Autodesk Inventor part; units mm, degrees
ref_plane "BoardFrontPlane" through (0, 0, 0) normal (0, 0, 1) x (1, 0, 0)
ref_plane "YZ Plane" through (0, 0, 0) normal (1, 0, 0) x (0, 1, 0)
ref_plane "XZ Plane" through (0, 0, 0) normal (0, 1, 0) x (-1, 0, 0)
ref_plane "BoardFrontPlane" through (0, 0, 0) normal (0, 0, 1) x (1, 0, 0)
sketch "Sketch1" plane through (0, 0, 0) normal (0, 0, 1) x (1, 0, 0)
  line L0 (35, 26) -> (35, 27)
  line L1 (35, 27) -> (75, 27)
  line L2 (75, 27) -> (75, 26)
  line L3 (75, 26) -> (83.3, 26)
  line L4 (83.3, 26) -> (83.3, 33.05)
  line L5 (83.3, 33.05) -> (128.7, 33.05)
  line L6 (128.7, 33.05) -> (128.7, 26)
  line L7 (128.7, 26) -> (147, 26)
  line L8 (147, 26) -> (147, 27)
  line L9 (147, 27) -> (171, 27)
  line L10 (171, 27) -> (171, 26)
  line L11 (171, 26) -> (186, 26)
  line L12 (186, 26) -> (186, 113)
  line L13 (186, 113) -> (128.7, 113)
  line L14 (128.7, 113) -> (128.7, 105.95)
  line L15 (128.7, 105.95) -> (83.3, 105.95)
  line L16 (83.3, 105.95) -> (83.3, 113)
  line L17 (83.3, 113) -> (26, 113)
  line L18 (26, 113) -> (26, 26)
  line L19 (26, 26) -> (35, 26)
extrude "BoardOutline" add sketch "Sketch1" along normal blind 1.5957
ref_plane "Work Plane2" through (106, 26, 0) normal (1, 0, 0) x (0, 0, -1)
ref_plane "Work Plane3" through (171, 69.5, 0) normal (0, -1, 0) x (1, 0, 0)
sketch "Sketch4" plane through (0, 0, 1.5957) normal (0, 0, 1) x (1, 0, 0)
  line L0 (83.3, 26) -> (83.3, 33.05)
  line L1 (83.3, 33.05) -> (128.7, 33.05)
  line L2 (128.7, 33.05) -> (128.7, 26)
  line L3 (26, 113) -> (26, 26)
  line L4 (83.3, 26) -> (128.7, 26)
  point P0 (83.3, 29.525)
  point P1 (186, 26)
  dimension "d9" = 57.3
  dimension "d10" = 57.3
  dimension "d11" = 7.05
sketch "Sketch8" plane through (0, 0, 1.5957) normal (0, 0, 1) x (1, 0, 0)
  point P0 (106, 94.5)
hole "Free-Hole1_1" at (106, 94.5, 1.5957) direction (0, 0, -1) diameter 3.6 end through all
sketch "Sketch9" plane through (0, 0, 1.5957) normal (0, 0, 1) x (1, 0, 0)
  point P0 (106, 44.5)
hole "Free-Hole1_2_1" at (106, 44.5, 1.5957) direction (0, 0, -1) diameter 3.6 end through all
sketch "Sketch11" plane through (0, 0, 1.5957) normal (0, 0, 1) x (1, 0, 0)
  point P0 (46, 94.5)
hole "Free-Hole4_1" at (46, 94.5, 1.5957) direction (0, 0, -1) diameter 3.6 end through all
sketch "Sketch12" plane through (0, 0, 1.5957) normal (0, 0, 1) x (1, 0, 0)
  point P0 (46, 44.5)
hole "Free-Hole4_2_1" at (46, 44.5, 1.5957) direction (0, 0, -1) diameter 3.6 end through all
sketch "Sketch13" plane through (0, 0, 1.5957) normal (0, 0, 1) x (1, 0, 0)
  point P0 (166, 44.5)
hole "Free-Hole4_3_1" at (166, 44.5, 1.5957) direction (0, 0, -1) diameter 3.6 end through all
sketch "Sketch14" plane through (0, 0, 1.5957) normal (0, 0, 1) x (1, 0, 0)
  point P0 (166, 94.5)
hole "Free-Hole4_4_1" at (166, 94.5, 1.5957) direction (0, 0, -1) diameter 3.6 end through all
sketch "img_Top" plane through (0, 0, 1.5957) normal (0, 0, 1) x (1, 0, 0)
  line L0 (26, 113) -> (186, 113) construction
  line L1 (186, 113) -> (186, 26.0021) construction
  line L2 (186, 26.0021) -> (26, 26.0021) construction
  line L3 (26, 26.0021) -> (26, 113) construction
decal "Decal_Top"
properties part number "ledbrick_plus_led_BOARD"
The listing builds one solid part. Answer for the finished solid, in the listing's coordinates (mm). Coordinates: 2 decimals unless noted, no trailing zeros. Write each loop counter-clockwise with the first axis right and the second up, starting at its lowest first coordinate (ties: lowest second). Pieces come first, ordered by that corner, then holes. Notation, with made-up numbers: (-38.75, 78) -> (-24.75, 78) arc R17 cw to (-24.75, 84) -> close; hole circle Ø4 at (72.25, 30.25). An arc over 180 degrees is marked (long way). Write each question's results on one line, items separated by ' | '. Start each with the question number.
1) For a pull along Y with two mould halves and no side action, classify faces 1 (the cylindrical face through (167.757, 94.89, 0.787)), 2 (the flat face through (105, 70, 1.596)) as +Y half, -Y half, draft (parallel to the pull), parting line (faces both ways), or undercut.
2) A cutting plane is placed at A-A (x = 166). Determine the outline of the cut face in (y, z).
3) A cutting plane is placed at D-D (x = 106). Determine the outline of the cut face in (y, z).
4) A cutting plane is placed at B-B (z = 0.4). Determine the outline of the cut face in (x, y), then the cut area to 3 significant figures.
5) Straight lines are drawn through the part: probe 1 along X at (y, z) = (94.5, 0.55); probe 2 along Y at (x, z) = (106, 1.1); probe 3 along Y at (x, z) = (46, 1.15). For each, find the intervals that lie inside material, in ascending order.
6) A cutting plane is placed at C-C (y = 44.5). Determine the outline of the cut face in (x, z).
7) Flat-ended cylindrical pins translate along their axes: pin 1 Ø0.5 at (x, z) = (97, 1) entering from +Y; pin 2 Ø0.8 at (x, z) = (116, 1) entering from -Y. Find the tip coordinate at first contact, or state that the pin passes through.
Values follow:
1) face 1: undercut | face 2: draft
2) outline: (27, 0) -> (42.7, 0) -> (42.7, 1.6) -> (27, 1.6) -> close; (46.3, 0) -> (92.7, 0) -> (92.7, 1.6) -> (46.3, 1.6) -> close; (96.3, 0) -> (113, 0) -> (113, 1.6) -> (96.3, 1.6) -> close
3) outline: (33.05, 0) -> (42.7, 0) -> (42.7, 1.6) -> (33.05, 1.6) -> close; (46.3, 0) -> (92.7, 0) -> (92.7, 1.6) -> (46.3, 1.6) -> close; (96.3, 0) -> (105.95, 0) -> (105.95, 1.6) -> (96.3, 1.6) -> close
4) outline: (26, 26) -> (35, 26) -> (35, 27) -> (75, 27) -> (75, 26) -> (83.3, 26) -> (83.3, 33.05) -> (128.7, 33.05) -> (128.7, 26) -> (147, 26) -> (147, 27) -> (171, 27) -> (171, 26) -> (186, 26) -> (186, 113) -> (128.7, 113) -> (128.7, 105.95) -> (83.3, 105.95) -> (83.3, 113) -> (26, 113) -> close; hole circle Ø3.6 at (46, 44.5); hole circle Ø3.6 at (46, 94.5); hole circle Ø3.6 at (106, 44.5); hole circle Ø3.6 at (106, 94.5); hole circle Ø3.6 at (166, 44.5); hole circle Ø3.6 at (166, 94.5) | area: 13,200 mm²
5) probe 1: 26 to 44.2, 47.8 to 104.2, 107.8 to 164.2, 167.8 to 186 | probe 2: 33.05 to 42.7, 46.3 to 92.7, 96.3 to 105.95 | probe 3: 27 to 42.7, 46.3 to 92.7, 96.3 to 113
6) outline: (26, 0) -> (44.2, 0) -> (44.2, 1.6) -> (26, 1.6) -> close; (47.8, 0) -> (104.2, 0) -> (104.2, 1.6) -> (47.8, 1.6) -> close; (107.8, 0) -> (164.2, 0) -> (164.2, 1.6) -> (107.8, 1.6) -> close; (167.8, 0) -> (186, 0) -> (186, 1.6) -> (167.8, 1.6) -> close
7) pin 1: y = 105.95 | pin 2: y = 33.05
